```python
from build123d import *

# Parameters (mm, degrees)
F0_R           = 5.334
F1_DEPTH       = 28.829
F2_R           = 13.271737
F3_DEPTH       = 25.4
F4_W           = 26.543474
F4_H           = 10.5664
F5_DEPTH       = 54.229
F6_W           = 8.128
F6_H           = 10.5664
F7_DEPTH       = 21.59
F9_DEPTH       = 21.59
F10_DEPTH      = 21.59
F11_R          = 1.5875
F12_DEPTH      = 5.334
F12_DEPTH_BACK = 5.334


with BuildPart() as f1:
    # F0 (on Front) → F1 (new body)
    with BuildSketch(Plane.XZ):
        Circle(F0_R)
    extrude(amount=F1_DEPTH)

    # F2 (on face) → F3 (join)
    with BuildSketch(Plane.XZ.offset(28.829)):
        Circle(F2_R)
    extrude(amount=F3_DEPTH)

    # F4 (on face) → F5 (intersect, through all)
    with BuildSketch(Plane.XZ.offset(54.229)):
        Rectangle(F4_W, F4_H)
    extrude(amount=-F5_DEPTH, mode=Mode.INTERSECT)

    # F6 (on face) → F7 (cut)
    with BuildSketch(Plane.XZ.offset(54.229)):
        Rectangle(F6_W, F6_H)
    extrude(amount=-F7_DEPTH, mode=Mode.SUBTRACT)

    # F8 (on face) → F9 (cut)
    with BuildSketch(Plane.XZ.offset(54.229)):
        with BuildLine():
            Line((4.826, 1.812324), (-4.826, 1.812324))
            ThreePointArc((-4.826, 1.812324), (-5.364815, 1.58914), (-5.588, 1.050324))
            Line((-5.588, 1.050324), (-5.588, -1.050324))
            ThreePointArc((-5.588, -1.050324), (-5.364815, -1.58914), (-4.826, -1.812324))
            Line((-4.826, -1.812324), (4.826, -1.812324))
            ThreePointArc((4.826, -1.812324), (5.364815, -1.58914), (5.588, -1.050324))
            Line((5.588, -1.050324), (5.588, 1.050324))
            ThreePointArc((5.588, 1.050324), (5.364815, 1.58914), (4.826, 1.812324))
        make_face()
    extrude(amount=-F9_DEPTH, mode=Mode.SUBTRACT)

    # F8 (on face) → F10 (cut)
    with BuildSketch(Plane.XZ.offset(54.229)):
        with BuildLine():
            Line((4.826, 1.812324), (-4.826, 1.812324))
            ThreePointArc((-4.826, 1.812324), (-5.364815, 1.58914), (-5.588, 1.050324))
            Line((-5.588, 1.050324), (-5.588, -1.050324))
            ThreePointArc((-5.588, -1.050324), (-5.364815, -1.58914), (-4.826, -1.812324))
            Line((-4.826, -1.812324), (4.826, -1.812324))
            ThreePointArc((4.826, -1.812324), (5.364815, -1.58914), (5.588, -1.050324))
            Line((5.588, -1.050324), (5.588, 1.050324))
            ThreePointArc((5.588, 1.050324), (5.364815, 1.58914), (4.826, 1.812324))
        make_face()
    extrude(amount=-F10_DEPTH, mode=Mode.SUBTRACT)

    # F11 (on Right) → F12 (cut, two sides)
    with BuildSketch(Plane.YZ) as f12_sk:
        with Locations((-6.3119, 0)):
            Circle(F11_R)
    extrude(amount=F12_DEPTH, mode=Mode.SUBTRACT)
    extrude(f12_sk.sketch, amount=-F12_DEPTH_BACK, mode=Mode.SUBTRACT)


solid = f1.part
```
Could you check a few things on this model? Use its own coordinates, in mm. A direction names the side the tool comes from. Give positions to 0.01 mm unless a question says otherwise; leave off trailing zeros. Loops run counter-clockwise (first coordinate to the right, second up) from the corner with the lowest first, then second, coordinate; pieces in that order, holes last. Notation, with made-up numbers: (-16, 45) - (-2, 45) arc R12 cw to (-2, 68) - close; hole circle Ø10 at (6, 76.5). An arc over 180 degrees is marked (long way). Use one line per item in the form item = value.
1. I want a section at C-C (x = -3). Please give me the cut outline in (y, z) (1 decimal), and give its area (3 significant figures).
Response values:
outline = (-32.6, -5.3) - (-28.8, -5.3) - (-28.8, -4.4) - (0, -4.4) - (0, 4.4) - (-28.8, 4.4) - (-28.8, 5.3) - (-32.6, 5.3) - close; hole circle Ø3.2 at (-6.3, 0)
area = 287 mm²
2. I want a section at A-A (z = 0). Please give me the cut outline in (x, y).
Response values:
outline = (-13.27, -54.23) - (-5.59, -54.23) - (-5.59, -32.64) - (5.59, -32.64) - (5.59, -54.23) - (13.27, -54.23) - (13.27, -28.83) - (5.33, -28.83) - (5.33, -7.9) - (-5.33, -7.9) - (-5.33, -28.83) - (-13.27, -28.83) - close; (-5.33, -4.72) - (5.33, -4.72) - (5.33, 0) - (-5.33, 0) - close
3. Thinking about a two-plate mould opening in X: for faces 6 (the face through (-4.064, -44, 4)), 7 (the face through (-13.27, -41.35, 0.08)), 8 (the face through (4.5, -39.3, 5.283)), 9 (the face through (-5.588, -44, 0)), which applies, released by +X, released by -X, zero draft, split by the parting line, or undercut?
Response values:
face_6 = undercut
face_7 = released by -X
face_8 = zero draft
face_9 = undercut
4. I'm going to push flat-ended pins straight in: pin 1 Ø5 at (x, z) = (-0.5, 1) entering from -Y; pin 2 Ø3 at (y, z) = (-40.5, -3) entering from -X; pin 3 Ø1 at (y, z) = (-40.5, 3) entering from +X. Where does each tip first touch, or does it pass through?
Response values:
pin_1 = -32.64
pin_2 = -13.19
pin_3 = 13.03
5. I need wall thicknesses on probe 1 along Y at (x, z) = (-2.95, 0); probe 2 along Y at (x, z) = (-8.5, 3); probe 3 along X at (y, z) = (-40.5, -1). Which ranges of each line are inside material? Lowest first, please.
Response values:
probe_1 = -32.64 to -7.9, -4.72 to 0
probe_2 = -54.23 to -28.83
probe_3 = -13.23 to -5.59, 5.59 to 13.23
6. I want a section at D-D (z = -2.75). Please give me the cut outline in (x, y).
Response values:
outline = (-12.98, -54.23) - (-4.06, -54.23) - (-4.06, -32.64) - (4.06, -32.64) - (4.06, -54.23) - (12.98, -54.23) - (12.98, -28.83) - (4.57, -28.83) - (4.57, 0) - (-4.57, 0) - (-4.57, -28.83) - (-12.98, -28.83) - close
7. On a 3-axis mill with a long thin cutter (end or side, diameter ignored), from which of +Z, -Z, +X, -X, +Y, -Y can I reach the whole of each face in a straight line? I mean faces 1 (the face through (-5.333, -14.213, 0.107)), 2 (the face through (4.064, -44, -4)), 3 (the face through (5.588, -44, 0)), 4 (the face through (5.333, -14.213, -0.107)), 5 (the face through (13.27, -41.35, -0.08)). Say none if no direction works.
Response values:
face_1 = -X, +Y
face_2 = +Z, -Z, -Y
face_3 = -Y
face_4 = +X, +Y
face_5 = +X, +Y, -Y
8. I want a section at B-B (y = -45.5). Please give me the cut outline in (x, z).
Response values:
outline = (-12.17, -5.28) - (-4.06, -5.28) - (-4.06, -1.81) - (-4.83, -1.81) arc R0.76 cw to (-5.59, -1.05) - (-5.59, 1.05) arc R0.76 cw to (-4.83, 1.81) - (-4.06, 1.81) - (-4.06, 5.28) - (-12.17, 5.28) arc R13.27 ccw to start; (4.06, -5.28) - (12.17, -5.28) arc R13.27 ccw to (12.17, 5.28) - (4.06, 5.28) - (4.06, 1.81) - (4.83, 1.81) arc R0.76 cw to (5.59, 1.05) - (5.59, -1.05) arc R0.76 cw to (4.83, -1.81) - (4.06, -1.81) - close
